Job drawing, mm, ordinate dimensions from the low corner. One solid piece. A direction names the side the tool comes from. Give positions to 0.01 mm unless a question says otherwise; leave off trailing zeros. Loops run counter-clockwise (first coordinate to the right, second up) from the corner with the lowest first, then second, coordinate; pieces in that order, holes last. Notation, with made-up numbers: (-3.75, 54.5) - (34.25, 54.5) arc R32 cw to (34.25, 83.5) - close; hole circle Ø5 at (-13, 29.5). An arc over 180 degrees is marked (long way). Use a Markdown table: item, result.
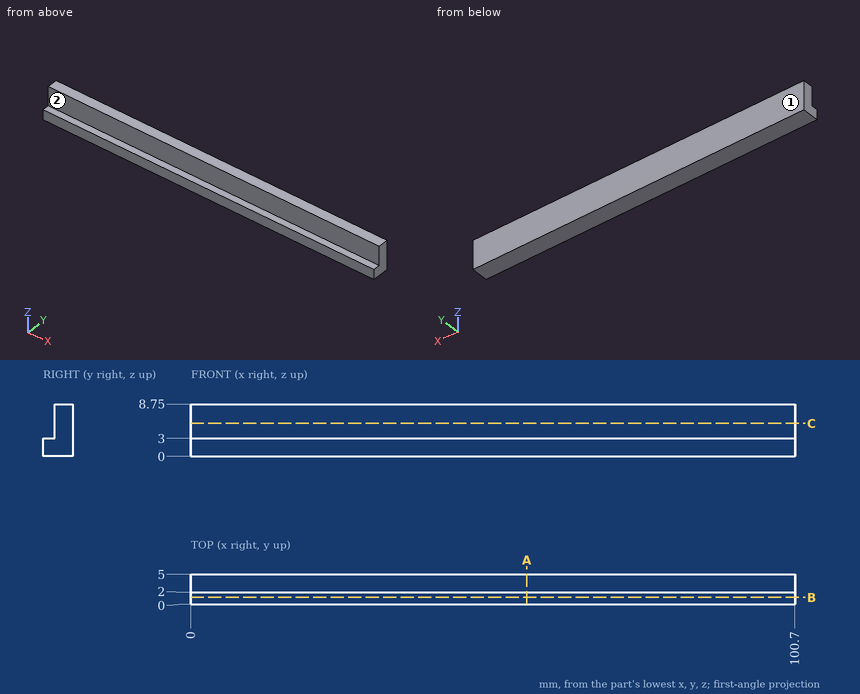
(1) Slice it at B-B, the plane y = 1.2. Write the cut outline in (x, z).
Computed:
| item | result |
|---|---|
| outline | (0, 0) - (100.7, 0) - (100.7, 3) - (0, 3) - close |
(2) Slice it at A-A, the plane x = 56. Write the cut outline in (y, z).
Computed:
| item | result |
|---|---|
| outline | (0, 0) - (5, 0) - (5, 8.75) - (2, 8.75) - (2, 3) - (0, 3) - close |
(3) Drill centre lines: probe 1 along Z at (x, y) = (26.5, 0.55); probe 2 along Y at (x, z) = (33.5, 3.75). Where is each one in solid material? Low to high. Write a range as [from, to].
Computed:
| item | result |
|---|---|
| probe 1 | [0, 3] |
| probe 2 | [2, 5] |
(4) Slice it at C-C, the plane z = 5.5. Write the cut outline in (x, y), plus the area to 3 significant figures.
Computed:
| item | result |
|---|---|
| outline | (0, 2) - (100.7, 2) - (100.7, 5) - (0, 5) - close |
| area | 302 mm² |
(5) Pin check, flat tip, straight feed: P1, Ø4, axis at x = 48.5, z = 7, coming from the -Y side. Stop position of the tip, or through.
Computed:
| item | result |
|---|---|
| P1 | y = 2 |
(6) 3-axis set-ups, long thin cutter, end or side, ignore diameter. For the marked faces 1 and 2: which of +Z, -Z, +X, -X, +Y, -Y reach the whole face in a straight line?
Computed:
| item | result |
|---|---|
| face 1 | +Z, -Z, +X, -X, +Y |
| face 2 | +Z, +X, -X, -Y |
